The figure shows three views and two pictorial views of one solid part (mm, origin at its lowest corner). Answer the questions. A direction names the side the tool comes from. Coordinates: 2 decimals unless noted, no trailing zeros. Loops run counter-clockwise (first coordinate to the right, second up) from the corner with the lowest first, then second, coordinate; pieces in that order, holes last. Notation, with made-up numbers: (74, 79.25) - (104, 79.25) arc R23 cw to (104, 107.25) - close; hole circle Ø6 at (15.5, -34). An arc over 180 degrees is marked (long way). Return JSON: item names as keys, results as strings. Group by question number.
1. Section A-A (x = 39) is taken. Write down the section's boundary in (y, z), and give its area (3 significant figures).
2. Section C-C (z = 18.5) is taken. Write down the section's boundary in (x, y), and give its area (3 significant figures).
3. Section B-B (x = 72.5) is taken. Write down the section's boundary in (y, z).
4. This flat-tipped pin is pushed along its axis until it touches: P1, Ø3, axis at y = 32, z = 3.5, coming from the -X side. Where does it stop, or does it pass through?
5. Find the intervals of material crossed by line 1 along X through (y, z) = (34.5, 13); line 2 along Y through (x, z) = (77, 5.25); line 3 along Y through (x, z) = (30.5, 4), in increasing order.
6. Section D-D (y = 55.5) is taken. Write down the section's boundary in (x, z).
7. Which of the six approach directions +Z, -Z, +X, -X, +Y, -Y give full straight-line access (tool end or side, diameter ignored) to the marked faces 5, 6 and 7?
8. The mould has two halves that part along Y. Classify the marked faces 1, 2, 3 and 4: pulls with the +Y half, pulls with the -Y half, needs draft (parallel to the pull), parting line crosses it, or undercut.
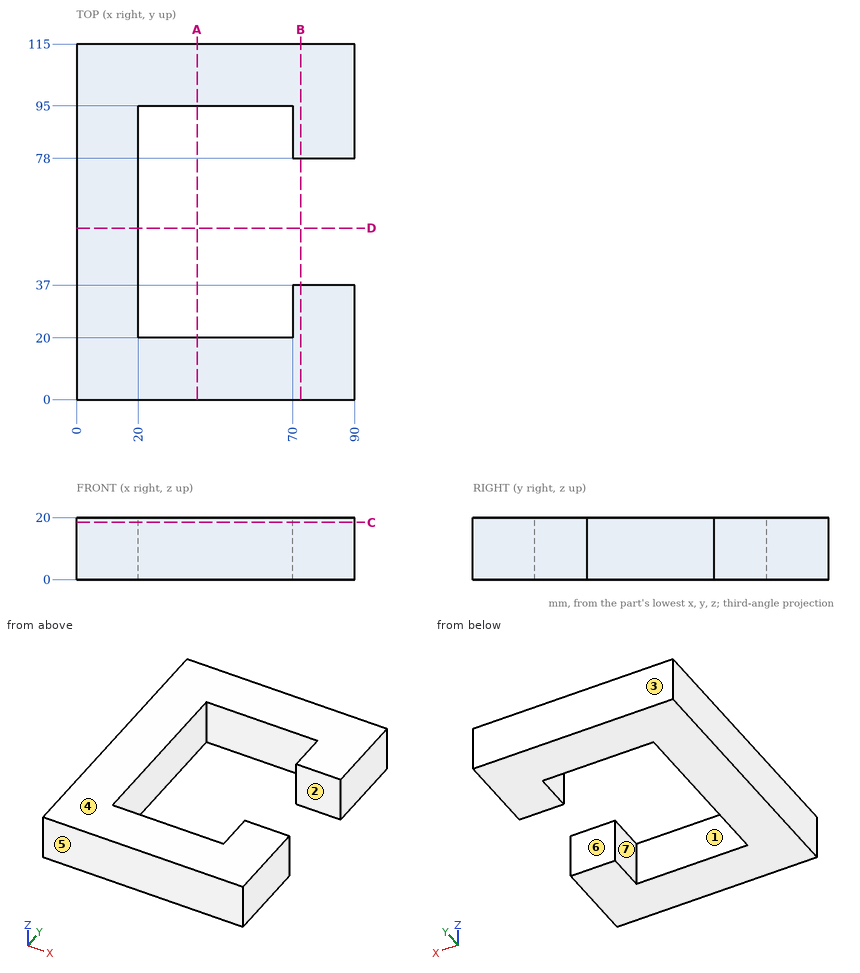
The answers:
{
 "1": {"outline": "(0, 0) - (20, 0) - (20, 20) - (0, 20) - close; (95, 0) - (115, 0) - (115, 20) - (95, 20) - close", "area": "800 mm2"},
 "2": {"outline": "(0, 0) - (90, 0) - (90, 37) - (70, 37) - (70, 20) - (20, 20) - (20, 95) - (70, 95) - (70, 78) - (90, 78) - (90, 115) - (0, 115) - close", "area": "5,780 mm2"},
 "3": {"outline": "(0, 0) - (37, 0) - (37, 20) - (0, 20) - close; (78, 0) - (115, 0) - (115, 20) - (78, 20) - close"},
 "4": {"P1": "stops at x = 0"},
 "5": {"line 1": "x = 0 to 20, 70 to 90", "line 2": "y = 0 to 37, 78 to 115", "line 3": "y = 0 to 20, 95 to 115"},
 "6": {"outline": "(0, 0) - (20, 0) - (20, 20) - (0, 20) - close"},
 "7": {"face 5": "+Z, -Z, +X, -X, -Y", "face 6": "+Z, -Z, +X", "face 7": "+Z, -Z"},
 "8": {"face 1": "undercut", "face 2": "undercut", "face 3": "pulls with the +Y half", "face 4": "needs draft"}
}
